Part model, mm, in its own coordinate system. A direction names the side the tool comes from. Coordinates: 2 decimals unless noted, no trailing zeros. Loops run counter-clockwise (first coordinate to the right, second up) from the corner with the lowest first, then second, coordinate; pieces in that order, holes last. Notation, with made-up numbers: M 65.5,66.5 L 115.5,66.5 A24 ccw 115.5,94.5 Z; hole C -20.75,-4 d2. An arc over 180 degrees is marked long. Use a Markdown table: item, result. Add a question column.
1) Band-saw the part on B-B (z = -84.5). List the corners of the cut face in (x, y).
2) Band-saw the part on A-A (x = 0). List the corners of the cut face in (y, z), plus the area to 3 significant figures.
3) Band-saw the part on D-D (x = 14.5). List the corners of the cut face in (y, z), plus the area to 3 significant figures.
4) Tool access for faces 5 (the flat face through (-4, 6, -71)), 6 (the cylindrical face through (0.352, 11.24, -89.272)), 7 (the flat face through (8, 10.5, -79)), 8 (the cylindrical face through (-10.25, 3.72, -2.28)): list every direction of +Z, -Z, +X, -X, +Y, -Y with a clear straight run to the whole face (end or side of a thin tool).
5) Pin check, flat tips, straight feed: pin 1 Ø17 at (x, z) = (-3, -78.5) entering from -Y; pin 2 Ø2 at (x, y) = (8.5, 3.5) entering from +Z; pin 3 Ø9.5 at (x, z) = (0, 0) entering from -Y; pin 4 Ø1.5 at (x, y) = (-10, 1.5) entering from +Z. Stop position of each tip, or through.
6) Wall check: probe 1 along X at (y, z) = (11.6, -81.28); probe 2 along X at (y, z) = (8.05, -81.28); probe 3 along Y at (x, z) = (7, -13). Give the ranges that are in metal, low to high. Write a range as from..to.
7) Band-saw the part on C-C (y = 3.5). List the corners of the cut face in (x, z).
8) Pull direction Z, two halves, no side cores. Call faces 1 (the flat face through (0, 6, -18)), 2 (the cylindrical face through (3.154, 8.218, -71.265)), 3 (the cylindrical face through (-7.81, 0.74, 1.73)), 4 (the flat face through (-0.236, 3.042, -50.316)): released by +Z, released by -Z, zero draft, split by the parting line, or undercut.
from build123d import *

# Parameters (mm, degrees)
SKETCH1_R           = 10.499999955
BOSS_EXTRUDE1_DEPTH = 12
SKETCH2_R           = 10.499999955
CUT_EXTRUDE1_DEPTH  = 6
BOSS_EXTRUDE2_START = -1.5
SKETCH3_R           = 10.499999955
SKETCH3_R_2         = 8
BOSS_EXTRUDE2_DEPTH = 1.5
CUT_EXTRUDE2_START  = -6
CUT_EXTRUDE2_DEPTH  = 6
SKETCH5_R           = 10.499999955
SKETCH5_R_2         = 8
BOSS_EXTRUDE3_DEPTH = 1.5
CUT_EXTRUDE6_DEPTH  = 105.447053023


with BuildPart() as part:
    # Sketch1 → Boss-Extrude1 (new body)
    with BuildSketch(Plane(origin=(0, 0, 0), x_dir=(1, 0, 0), z_dir=(0, 1, 0))):
        with BuildLine():
            Line((-16.849999955, 0), (-16.849999955, 81.28))
            ThreePointArc((-16.849999955, 81.28), (0, 98.129999955), (16.849999955, 81.28))
            Line((16.849999955, 81.28), (16.849999955, 0))
            ThreePointArc((16.849999955, 0), (0, -16.849999955), (-16.849999955, 0))
        make_face()
        with Locations(Location((0, 0, 0), (0, 0, 270))):
            Circle(SKETCH1_R, mode=Mode.SUBTRACT)
        with Locations(Location((0, 81.28, 0), (0, 0, 270))):
            Circle(SKETCH1_R, mode=Mode.SUBTRACT)
    extrude(amount=BOSS_EXTRUDE1_DEPTH)

    # Sketch2 → Cut-Extrude1 (cut)
    with BuildSketch(Plane.XZ):
        with BuildLine():
            Line((-16.849999955, -60.96), (-16.849999955, -81.28))
            ThreePointArc((-16.849999955, -81.28), (0, -98.129999955), (16.849999955, -81.28))
            Line((16.849999955, -81.28), (16.849999955, -60.96))
            Line((16.849999955, -60.96), (-16.849999955, -60.96))
        make_face()
        with Locations(Location((0, -81.28, 0), (0, 0, 270))):
            Circle(SKETCH2_R, mode=Mode.SUBTRACT)
    extrude(amount=-CUT_EXTRUDE1_DEPTH, mode=Mode.SUBTRACT)

    # Sketch3 → Boss-Extrude2 (add)
    with BuildSketch(Plane(origin=(0, 12, 0), x_dir=(1, 0, 0), z_dir=(0, 1, 0)).offset(BOSS_EXTRUDE2_START)):
        with Locations(Location((0, 81.28, 0), (0, 0, 90))):
            Circle(SKETCH3_R)
        with Locations(Location((0, 81.28, 0), (0, 0, 270))):
            Circle(SKETCH3_R_2, mode=Mode.SUBTRACT)
    extrude(amount=BOSS_EXTRUDE2_DEPTH)

    # Sketch4 → Cut-Extrude2 (cut)
    with BuildSketch(Plane(origin=(0, 12, 0), x_dir=(1, 0, 0), z_dir=(0, 1, 0)).offset(CUT_EXTRUDE2_START)):
        with BuildLine():
            Line((-16.849999955, 0), (-16.849999955, 20.32))
            Line((-16.849999955, 20.32), (16.849999955, 20.32))
            Line((16.849999955, 20.32), (16.849999955, 0))
            ThreePointArc((16.849999955, 0), (0, -16.849999955), (-16.849999955, 0))
        make_face()
    extrude(amount=CUT_EXTRUDE2_DEPTH, mode=Mode.SUBTRACT)

    # Sketch5 → Boss-Extrude3 (add)
    with BuildSketch(Plane.XZ):
        with Locations(Location((0, 0, 0), (0, 0, 270))):
            Circle(SKETCH5_R)
        with Locations(Location((0, 0, 0), (0, 0, 270))):
            Circle(SKETCH5_R_2, mode=Mode.SUBTRACT)
    extrude(amount=-BOSS_EXTRUDE3_DEPTH)

    # Sketch8 → Cut-Extrude6 (cut, through all)
    with BuildSketch(Plane(origin=(-16.849999955, 0, 0), x_dir=(0, 0, -1), z_dir=(1, 0, 0))):
        Polygon((20.32, 6), (39.37, 6), (60.96, 12), (20.32, 12), align=None)
        Polygon((60.96, 6), (39.37, 0), (60.96, 0), align=None)
    extrude(amount=CUT_EXTRUDE6_DEPTH, mode=Mode.SUBTRACT)


solid = part.part
Entries:
| question | item | result |
|---|---|---|
| 1 | outline | M -16.54,6 L -9.99,6 L -9.99,10.5 L -7.32,10.5 L -7.32,12 L -16.54,12 Z; M 7.32,10.5 L 9.99,10.5 L 9.99,6 L 16.54,6 L 16.54,12 L 7.32,12 Z |
| 2 | outline | M 0,-39.37 L 6,-60.96 L 6,-70.78 L 10.5,-70.78 L 10.5,-73.28 L 12,-73.28 L 12,-60.96 L 6,-39.37 L 6,-10.5 L 1.5,-10.5 L 1.5,-8 L 0,-8 Z; M 0,8 L 1.5,8 L 1.5,10.5 L 6,10.5 L 6,16.85 L 0,16.85 Z; M 6,-98.13 L 12,-98.13 L 12,-89.28 L 10.5,-89.28 L 10.5,-91.78 L 6,-91.78 Z |
| 2 | area | 453 mm2 |
| 3 | outline | M 0,-39.37 L 6,-60.96 L 6,-89.86 L 12,-89.86 L 12,-60.96 L 6,-39.37 L 6,8.58 L 0,8.58 Z |
| 3 | area | 591 mm2 |
| 4 | face 5 | -Z, +X, -X, -Y |
| 4 | face 6 | +Y, -Y |
| 4 | face 7 | -Y |
| 4 | face 8 | +Y |
| 5 | pin 1 | y = 6 |
| 5 | pin 2 | z = 15.09 |
| 5 | pin 3 | through |
| 5 | pin 4 | z = 14.08 |
| 6 | probe 1 | -16.85..-8, 8..16.85 |
| 6 | probe 2 | -16.85..-10.5, 10.5..16.85 |
| 6 | probe 3 | 0..6 |
| 7 | outline | M -16.85,-51.96 L 16.85,-51.96 L 16.85,0 A16.85 ccw -16.85,0 Z; hole C 0,0 d21 |
| 8 | face 1 | zero draft |
| 8 | face 2 | undercut |
| 8 | face 3 | undercut |
| 8 | face 4 | released by -Z |
